Could you check a few things on this model? Use its own coordinates, in mm. Face numbers are marked on the shaded views. A direction names the side the tool comes from. Coordinates: 2 decimals unless noted, no trailing zeros. Write each loop counter-clockwise with the first axis right and the second up, starting at its lowest first coordinate (ties: lowest second). Pieces come first, ordered by that corner, then holes.
Item 1: For P1, Ø6, axis at y = 46.5, z = -14.5, coming from the +X side; P2, Ø4, axis at y = 38.1, z = -12.7, coming from the +X side, each with a flat end and sliding along its axis, tell me the tip position at first contact or that it passes through.
Item 2: I want a section at A-A on y = 12.7. Please give me the cut outline in (x, z).
Item 3: I want a section at D-D on y = 76.2. Please give me the cut outline in (x, z) (1 decimal), then the cut area to 3 significant figures.
Item 4: If I drill on probe 1 along Y at (x, z) = (1.25, -12.7); probe 2 along Z at (x, y) = (8.25, 4); probe 3 along X at (y, z) = (57, -17.5), over which ranges is the centre line in solid material (lowest first)?
Item 5: I want a section at C-C on z = -12.7. Please give me the cut outline in (x, y).
Item 6: I want a section at B-B on x = 12.7. Please give me the cut outline in (y, z) (1 decimal).
Item 7: Which directions (+Z, -Z, +X, -X, +Y, -Y) give clear straight access to the entire face, cutting with the end or side of a thin tool? Please do the marked faces 1 and 2.
from build123d import *

# Parameters (mm, degrees)
BOSS_EXTRUDE1_DEPTH = 88.9
SKETCH2_R           = 2.54
CUT_EXTRUDE1_DEPTH  = 88.9
SKETCH3_R           = 3.175
CUT_EXTRUDE2_DEPTH  = 88.9


with BuildPart() as part:
    # Sketch1 → Boss-Extrude1 (new body)
    with BuildSketch(Plane(origin=(0, 0, 0), x_dir=(1, 0, 0), z_dir=(0, 1, 0))):
        Polygon((0, 0), (0, 25.4), (1.5875, 25.4), (1.5875, 1.5875), (25.4, 1.5875), (25.4, 0), align=None)
    extrude(amount=BOSS_EXTRUDE1_DEPTH)

    # Sketch2 → Cut-Extrude1 (cut)
    with BuildSketch(Plane.ZY):
        with Locations((-12.7, 38.1)):
            Circle(SKETCH2_R)
        with Locations((-12.7, 12.7)):
            Circle(SKETCH2_R)
    extrude(amount=-CUT_EXTRUDE1_DEPTH, mode=Mode.SUBTRACT)

    # Sketch3 → Cut-Extrude2 (cut)
    with BuildSketch(Plane(origin=(0, 0, -1.5875), x_dir=(-1, 0, 0), z_dir=(0, 0, -1))):
        with Locations((-12.7, 76.2)):
            Circle(SKETCH3_R)
    extrude(amount=-CUT_EXTRUDE2_DEPTH, mode=Mode.SUBTRACT)


solid = part.part
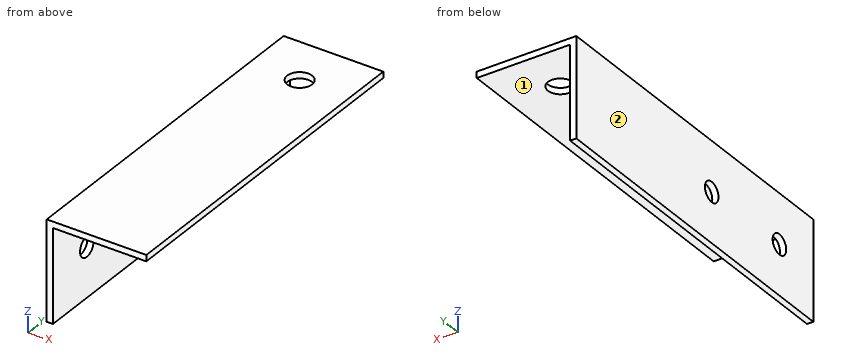
Response values:
1. P1: stops at x = 1.59
1. P2: passes through
2. outline: (0, -25.4) - (1.59, -25.4) - (1.59, -15.24) - (0, -15.24) - close; (0, -10.16) - (1.59, -10.16) - (1.59, -1.59) - (25.4, -1.59) - (25.4, 0) - (0, 0) - close
3. outline: (0, -25.4) - (1.6, -25.4) - (1.6, -1.6) - (9.5, -1.6) - (9.5, 0) - (0, 0) - close; (15.9, -1.6) - (25.4, -1.6) - (25.4, 0) - (15.9, 0) - close
3. area: 68.0 mm2
4. probe 1: y = 0 to 10.16, 15.24 to 35.56, 40.64 to 88.9
4. probe 2: z = -1.59 to 0
4. probe 3: x = 0 to 1.59
5. outline: (0, 0) - (1.59, 0) - (1.59, 10.16) - (0, 10.16) - close; (0, 15.24) - (1.59, 15.24) - (1.59, 35.56) - (0, 35.56) - close; (0, 40.64) - (1.59, 40.64) - (1.59, 88.9) - (0, 88.9) - close
6. outline: (0, -1.6) - (73, -1.6) - (73, 0) - (0, 0) - close; (79.4, -1.6) - (88.9, -1.6) - (88.9, 0) - (79.4, 0) - close
7. face 1: -Z, +X, +Y, -Y
7. face 2: +Z, -Z, -X, +Y, -Y
